Build history of the part. All positions in model axes, mm. Round coordinates to 2 decimals unless told otherwise and drop trailing zeros. Write each loop counter-clockwise with the first axis right and the second up, starting at its lowest first coordinate (ties: lowest second). Pieces come first, ordered by that corner, then holes. Notation, with made-up numbers: (79, 1) -> (118, 1) arc R20 cw to (118, 23) -> close; hole circle Ø7 at (-13.5, 42). An arc over 180 degrees is marked (long way). Answer as CSV lines item,"result".
from build123d import *

# Parameters (mm, degrees)
SKETCH_1_W             = 525
SKETCH_1_H             = 5
SM_BASE_FLANGE_1_DEPTH = 50
SKETCH_6_R             = 5.5
CUT_EXTRUDE_1_DEPTH    = 10
CUT_EXTRUDE_2_DEPTH    = 10
SKETCH_8_R             = 6.5
CUT_EXTRUDE_3_DEPTH    = 10
OTHER_START            = -5
OTHER_1_DEPTH          = 5


# Read off the part's stored shape, not the designer's step: Затупленный угол1
# Sheet-metal steps are written as plain solids
with BuildPart() as part:
    # Sketch 1 → Базовая кромка1 (new body)
    with BuildSketch(Plane.XY):
        with Locations((55.681818182, -2.5)):
            Rectangle(SKETCH_1_W, SKETCH_1_H)
    extrude(amount=SM_BASE_FLANGE_1_DEPTH)

    # Эскиз6 → Вырез-Вытянуть1 (cut)
    with BuildSketch(Plane(origin=(0, 0, 0), x_dir=(1, 0, 0), z_dir=(0, 1, 0))):
        with Locations(Location((-191.818181818, -25, 0), (0, 0, 270))):
            Circle(SKETCH_6_R)
        with Locations(Location((-166.818181818, -25, 0), (0, 0, 270))):
            Circle(SKETCH_6_R)
    extrude(amount=-CUT_EXTRUDE_1_DEPTH, mode=Mode.SUBTRACT)

    # Эскиз7 → Вырез-Вытянуть2 (cut)
    with BuildSketch(Plane(origin=(0, 0, 0), x_dir=(1, 0, 0), z_dir=(0, 1, 0))):
        with BuildLine():
            Line((197.681818182, -19), (210.681818182, -19))
            ThreePointArc((210.681818182, -19), (216.681818182, -25), (210.681818182, -31))
            Line((210.681818182, -31), (197.681818182, -31))
            ThreePointArc((197.681818182, -31), (191.681818182, -25), (197.681818182, -19))
        make_face()
    extrude(amount=-CUT_EXTRUDE_2_DEPTH, mode=Mode.SUBTRACT)

    # Эскиз8 → Вырез-Вытянуть3 (cut)
    with BuildSketch(Plane(origin=(0, 0, 0), x_dir=(1, 0, 0), z_dir=(0, 1, 0))):
        with Locations(Location((298.181818182, -25, 0), (0, 0, 270))):
            Circle(SKETCH_8_R)
    extrude(amount=-CUT_EXTRUDE_3_DEPTH, mode=Mode.SUBTRACT)

    # Other 1 outline → Other 1 (cut)
    with BuildSketch(Plane(origin=(0, 0, 0), x_dir=(1, 0, 0), z_dir=(0, 1, 0)).offset(OTHER_START)):
        Polygon((318.181818182, 0), (313.181818182, 0), (318.181818182, -5), align=None)
        Polygon((-206.818181818, -5), (-201.818181818, 0), (-206.818181818, 0), align=None)
        Polygon((318.181818182, -50), (318.181818182, -45), (313.181818182, -50), align=None)
        Polygon((-201.818181818, -50), (-206.818181818, -45), (-206.818181818, -50), align=None)
    extrude(amount=OTHER_1_DEPTH, mode=Mode.SUBTRACT)


solid = part.part
1. Cut at B-B, the plane y = -1.55. Write the cut outline in (x, z), then the cut area to 3 significant figures.
Results found:
outline,"(-206.82, 5) -> (-201.82, 0) -> (313.18, 0) -> (318.18, 5) -> (318.18, 45) -> (313.18, 50) -> (-201.82, 50) -> (-206.82, 45) -> close; hole circle Ø11 at (-191.82, 25); hole circle Ø11 at (-166.82, 25); hole (197.68, 19) -> (210.68, 19) arc R6 ccw to (210.68, 31) -> (197.68, 31) arc R6 ccw to start; hole circle Ø13 at (298.18, 25)"
area,"25,600 mm2"
2. Probe line 1 along X through (y, z) = (-2.1, 25); line 2 along X through (y, z) = (-1.1, 23); line 3 along X through (y, z) = (-3.4, 48). List the from-to ranges inside material, lowest first.
Results found:
line 1,"x = -206.82 to -197.32, -186.32 to -172.32, -161.32 to 191.68, 216.68 to 291.68, 304.68 to 318.18"
line 2,"x = -206.82 to -196.94, -186.69 to -171.94, -161.69 to 192.02, 216.34 to 292, 304.37 to 318.18"
line 3,"x = -203.82 to 315.18"
3. Cut at A-A, the plane z = 25. Write the cut outline in (x, y), then the cut area to 4 significant figures.
Results found:
outline,"(-206.82, -5) -> (-197.32, -5) -> (-197.32, 0) -> (-206.82, 0) -> close; (-186.32, -5) -> (-172.32, -5) -> (-172.32, 0) -> (-186.32, 0) -> close; (-161.32, -5) -> (191.68, -5) -> (191.68, 0) -> (-161.32, 0) -> close; (216.68, -5) -> (291.68, -5) -> (291.68, 0) -> (216.68, 0) -> close; (304.68, -5) -> (318.18, -5) -> (318.18, 0) -> (304.68, 0) -> close"
area,"2,325 mm2"
4. Mould opens along Z. For faces 1 (the cylindrical face through (-161.365, -2.465, 24.284)), 2 (the flat face through (52, 0, 25)) say: +Z half, -Z half, draft (parallel to the pull), parting line (faces both ways), or undercut.
Results found:
face 1,"undercut"
face 2,"draft"
